The listing builds one solid part. Answer for the finished solid, in the listing's coordinates (mm). A direction names the side the tool comes from. Give positions to 0.01 mm unless a question says otherwise; leave off trailing zeros. Order: outer loops, then holes, each group sorted by start corner. A loop starts at its lowest first (then second) coordinate and runs counter-clockwise, first axis right, second up. Notation, with made-up numbers: (24, -3.75) -> (46, -3.75) arc R35 cw to (46, 30.25) -> close; hole circle Ø11 at (36, 79.25). An arc over 180 degrees is marked (long way). Answer as a JSON object with one key per item and string values. Group by question number.
```python
from build123d import *

# Parameters (mm, degrees)
KREISMUSTER1_COUNT                 = 2
M8_GEWINDEBOHRUNG1_REACH           = 179.8
M8_GEWINDEBOHRUNG1_BORE_R          = 3.4
M8_GEWINDEBOHRUNG1_ON_FACE_2_REACH = 179.8
M8_GEWINDEBOHRUNG1_BORE_2_R        = 3.4


with BuildPart() as part:
    # Skizze1 → Rotation1 (revolve)
    with BuildSketch(Plane.XY, mode=Mode.PRIVATE) as rotation1_sk:
        with BuildLine():
            Line((0, 88.9), (278.4, 88.9))
            Line((278.4, 88.9), (278.4, 48.6))
            Line((278.4, 48.6), (258.4, 48.6))
            Line((258.4, 48.6), (258.4, 45))
            Line((258.4, 45), (226, 45))
            Line((226, 45), (226, 66.5))
            ThreePointArc((226, 66.5), (225.707106781, 67.207106781), (225, 67.5))
            Line((225, 67.5), (0, 67.5))
            Line((0, 67.5), (0, 88.9))
        make_face()
    revolve(rotation1_sk.sketch.rotate(Axis((0, 0, 0), (1, 0, 0)), 90), axis=Axis((0, 0, 0), (1, 0, 0)))  # turned: the seam where the file's is

    # Skizze6 → Schnitt-Rotation1 (revolve, cut)
    with BuildSketch(Plane.XY, mode=Mode.PRIVATE) as schnitt_rotation1_sk:
        Polygon((243.4, 88.9), (246.15, 88.9), (246.15, 69.3), (243.4, 67.647633298), align=None)
    schnitt_rotation1 = revolve(schnitt_rotation1_sk.sketch.rotate(Axis((243.4, 88.9, 0), (0, -1, 0)), 90), axis=Axis((243.4, 88.9, 0), (0, -1, 0)), mode=Mode.SUBTRACT)  # turned: the seam where the file's is

    # Kreismuster1: Schnitt-Rotation1 ×2 about axis
    kreismuster1_axis = Axis((0, 0, 0), (-1, 0, 0))
    for i in range(1, KREISMUSTER1_COUNT):
        add(schnitt_rotation1.rotate(kreismuster1_axis, i * 360 / KREISMUSTER1_COUNT), mode=Mode.SUBTRACT)

    # M8 Gewindebohrung1 bore (on position points) → M8 Gewindebohrung1 (cut, up to next)
    with BuildSketch(Plane(origin=(9, 88.9, 0), x_dir=(0, 0, 1), z_dir=(0, 1, 0)), mode=Mode.PRIVATE) as m8_gewindebohrung1_sk1:
        Circle(M8_GEWINDEBOHRUNG1_BORE_R)
    m8_gewindebohrung1_tool1 = extrude(m8_gewindebohrung1_sk1.sketch, amount=-M8_GEWINDEBOHRUNG1_REACH, mode=Mode.PRIVATE) & part.part
    add(m8_gewindebohrung1_tool1.solids().sort_by_distance((9, 88.9, 0))[0], mode=Mode.SUBTRACT)

    # M8 Gewindebohrung1 bore 2 (on position points) → M8 Gewindebohrung1 on face 2 (cut, up to next)
    with BuildSketch(Plane(origin=(9, 0, -88.9), x_dir=(-1, 0, 0), z_dir=(0, 0, -1)), mode=Mode.PRIVATE) as m8_gewindebohrung1_on_face_2_sk1:
        Circle(M8_GEWINDEBOHRUNG1_BORE_2_R)
    m8_gewindebohrung1_on_face_2_tool1 = extrude(m8_gewindebohrung1_on_face_2_sk1.sketch, amount=-M8_GEWINDEBOHRUNG1_ON_FACE_2_REACH, mode=Mode.PRIVATE) & part.part
    add(m8_gewindebohrung1_on_face_2_tool1.solids().sort_by_distance((9, 0, -88.9))[0], mode=Mode.SUBTRACT)


solid = part.part
```
(1) A cutting plane is placed at B-B (x = 204). Determine the outline of the cut face in (y, z), and give its area (3 significant figures).
(2) For a pull along Z with two mould halves and no side action, classify faces 1 (the cylindrical face through (141.149, -60.083, -65.523)), 2 (the cylindrical face through (5.68, 78.31, -0.74)), 3 (the flat face through (0, -66.3, 13.6)) as +Z half, -Z half, draft (parallel to the pull), parting line (faces both ways), or undercut.
(3) Which of the six approach directions +Z, -Z, +X, -X, +Y, -Y give full straight-line access (tool end or side, diameter ignored) to faces 4 (the cylindrical face through (268.26, -14.598, 46.356)), 5 (the flat face through (278.4, 38, 38)), 6 (the cylindrical face through (5.757, 1.021, -78.308)), 7 (the cylindrical face through (241.973, 39.923, 20.765)), 8 (the flat face through (226, 14, -43))?
(4) A cutting plane is placed at A-A (y = 0). Determine the outline of the cut face in (x, z), and give its area (3 significant figures).
(5) Find the intervals of material crossed by line 1 along X through (y, z) = (0, -75.75); line 2 along X through (y, z) = (84.25, 0); line 3 along Y through (x, z) = (267, 0), in increasing order. Write a range as [from, to].
(6) Flat-ended cylindrical pins translate along their axes: pin 1 Ø6 at (x, z) = (243.5, -15.5) entering from +Y; pin 2 Ø4 at (y, z) = (-3.5, -64) entering from -X; pin 3 Ø10 at (x, z) = (103, -34) entering from +Y. Find the tip coordinate at first contact, or state that the pin passes through.
Check sheet entries:
{
 "1": {"outline": "circle Ø177.8 at (0, 0); hole circle Ø135 at (0, 0)", "area": "10,500 mm2"},
 "2": {"face 1": "parting line", "face 2": "undercut", "face 3": "draft"},
 "3": {"face 4": "+X", "face 5": "+Z, -Z, +X, +Y, -Y", "face 6": "-Z", "face 7": "+X, -X", "face 8": "-X"},
 "4": {"outline": "(0, -88.9) -> (5.6, -88.9) -> (5.6, -67.5) -> (0, -67.5) -> close; (0, 67.5) -> (225, 67.5) arc R1 cw to (226, 66.5) -> (226, 45) -> (258.4, 45) -> (258.4, 48.6) -> (278.4, 48.6) -> (278.4, 88.9) -> (0, 88.9) -> close; (12.4, -88.9) -> (278.4, -88.9) -> (278.4, -48.6) -> (258.4, -48.6) -> (258.4, -45) -> (226, -45) -> (226, -66.5) arc R1 cw to (225, -67.5) -> (12.4, -67.5) -> close", "area": "14,000 mm2"},
 "5": {"line 1": "x = [0, 5.6], [12.4, 278.4]", "line 2": "x = [0, 5.6], [12.4, 240.65], [246.15, 278.4]", "line 3": "y = [-88.9, -48.6], [48.6, 88.9]"},
 "6": {"pin 1": "stops at y = 88.02", "pin 2": "stops at x = 226", "pin 3": "stops at y = 84.04"}
}
